Autodesk Inventor part; units mm, degrees
ref_plane "YZ Plane" through (0, 0, 0) normal (1, 0, 0) x (0, 1, 0)
ref_plane "XZ Plane" through (0, 0, 0) normal (0, 1, 0) x (-1, 0, 0)
ref_plane "XY Plane" through (0, 0, 0) normal (0, 0, 1) x (1, 0, 0)
sketch "Sketch1" plane through (0, 0, 0) normal (0, 0, 1) x (1, 0, 0)
  line L0 (-30, -40.5) -> (-30, 40.5)
  line L1 (-30, 40.5) -> (30, 40.5)
  line L2 (30, 40.5) -> (30, -40.5)
  line L3 (30, -40.5) -> (-30, -40.5)
  line L4 (-30, -40.5) -> (30, 40.5) construction
  line L5 (-30, 40.5) -> (30, -40.5) construction
  line L6 (-30, 40.5) -> (-10, 40.5)
  line L7 (-10, 40.5) -> (-10, 43.5)
  line L8 (-10, 43.5) -> (-30, 43.5)
  line L9 (-30, 43.5) -> (-30, 40.5) construction
  line L10 (30, 40.5) -> (10, 40.5)
  line L11 (10, 40.5) -> (10, 43.5)
  line L12 (10, 43.5) -> (30, 43.5)
  line L13 (30, 43.5) -> (30, 40.5)
  line L14 (-45.6, 0) -> (42.6, 0)
  line L15 (0, -60.9) -> (0, 60.9)
  line L16 (-10, -40.5) -> (-10, -43.5)
  line L17 (-10, -43.5) -> (-30, -43.5)
  line L18 (-30, -43.5) -> (-30, -40.5) construction
  line L19 (10, -40.5) -> (10, -43.5)
  line L20 (10, -43.5) -> (30, -43.5)
  line L21 (30, -43.5) -> (30, -40.5)
  line L22 (-30, -40.5) -> (-30, -24.3)
  line L23 (-30, -24.3) -> (-33, -24.3)
  line L24 (-33, -24.3) -> (-33, -40.5)
  line L25 (-33, -40.5) -> (-30, -40.5) construction
  line L26 (-30, -8.1) -> (-30, 8.1)
  line L27 (-30, 8.1) -> (-33, 8.1)
  line L28 (-33, 8.1) -> (-33, -8.1)
  line L29 (-33, -8.1) -> (-30, -8.1)
  line L30 (-30, 40.5) -> (-30, 24.3)
  line L31 (-30, 24.3) -> (-33, 24.3)
  line L32 (-33, 24.3) -> (-33, 40.5)
  line L33 (-33, 40.5) -> (-30, 40.5) construction
  line L34 (-30, 43.5) -> (-33, 43.5)
  line L35 (-33, 43.5) -> (-33, 40.5)
  line L36 (-30, -43.5) -> (-33, -43.5)
  line L37 (-33, -43.5) -> (-33, -40.5)
  point P0 (0, 0)
  point P1 (20, 43.5)
  point P2 (-20, 43.5)
  point P3 (20, -43.5)
  point P4 (-20, -43.5)
  point P5 (-33, 32.4)
  point P6 (-33, 0)
  point P7 (-33, -32.4)
  point P8 (-30, 0)
  dimension "d0" = 81
  dimension "d1" = 60
  dimension "d4" = 20
  dimension "d5" = 20
  dimension "d6" = 3
  dimension "d7" = 3
  dimension "d8" = 16.2
extrude "Extrusion1" add sketch "Sketch1" along normal blind 3
sketch "Sketch2" plane through (0, 0, 3) normal (0, 0, 1) x (1, 0, 0)
  line L0 (-45.6, 0) -> (42.6, 0)
  line L1 (0, -60.9) -> (0, 60.9)
  circle A0 centre (15, 0) radius 3.05
  line L2 (30, -43.5) -> (30, 43.5)
  dimension "d9" = 6.1
  dimension "d12" = 15
extrude "Extrusion2" cut sketch "Sketch2" against normal through all
equation "\"d4\" = 0.333333 * d1"
equation "\"d5\" = d4"
equation "\"d6\" = d2"
equation "\"d7\" = d2"
equation "\"d8\" = 0.2 * d0"
properties part number "top switch"
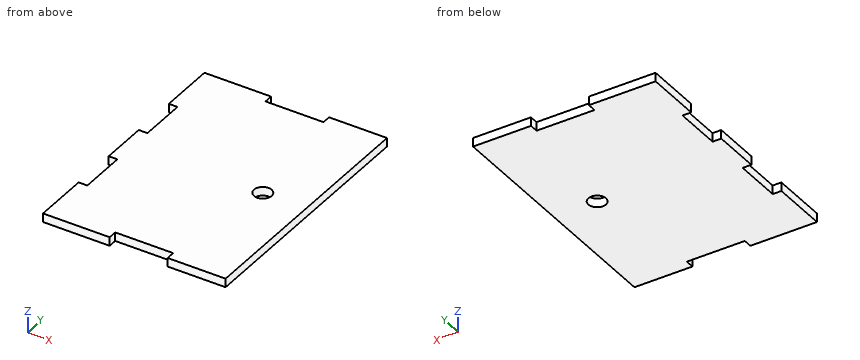
The listing builds one solid part. Answer for the finished solid, in the listing's coordinates (mm). Coordinates: 2 decimals unless noted, no trailing zeros. Write each loop counter-clockwise with the first axis right and the second up, starting at its lowest first coordinate (ties: lowest second). Pieces come first, ordered by that corner, then holes. Notation, with made-up numbers: M 86,-39.5 L 124,-39.5 A35 ccw 124,-5.5 Z; hole C 83.5,48 d10. An arc over 180 degrees is marked long. Put each result on its own line as item: value. Start each with the question number.
1. Consider line 1 (Y direction, x = 15, z = 2.15); line 2 (X direction, y = 0, z = 2); line 3 (Y direction, x = 0.5, z = 2.3). Determine where each line is inside the solid, lowest interval first. Write a range as from..to.
2. A cutting plane is placed at D-D on y = -18.5. Write down the section's boundary in (x, z), then the cut area to 3 significant figures.
3. A cutting plane is placed at B-B on y = 0. Write down the section's boundary in (x, z).
4. A cutting plane is placed at C-C on z = 1.85. Write down the section's boundary in (x, y), then the cut area to 3 significant figures.
5. A cutting plane is placed at A-A on x = 15. Write down the section's boundary in (y, z).
6. Flat-ended cylindrical pins translate along their axes: P1, Ø10, axis at x = 15, y = 0, coming from the +Z side; P2, Ø1.5, axis at y = 17, z = 1.5, coming from the -X side; P3, Ø1, axis at x = 4.5, z = 2.5, coming from the -Y side. Find the tip coordinate at first contact, or state that the pin passes through.
Resolved:
1. line 1: y = -43.5..-3.05, 3.05..43.5
1. line 2: x = -33..11.95, 18.05..30
1. line 3: y = -40.5..40.5
2. outline: M -30,0 L 30,0 L 30,3 L -30,3 Z
2. area: 180 mm2
3. outline: M -33,0 L 11.95,0 L 11.95,3 L -33,3 Z; M 18.05,0 L 30,0 L 30,3 L 18.05,3 Z
4. outline: M -33,-43.5 L -10,-43.5 L -10,-40.5 L 10,-40.5 L 10,-43.5 L 30,-43.5 L 30,43.5 L 10,43.5 L 10,40.5 L -10,40.5 L -10,43.5 L -33,43.5 L -33,24.3 L -30,24.3 L -30,8.1 L -33,8.1 L -33,-8.1 L -30,-8.1 L -30,-24.3 L -33,-24.3 Z; hole C 15,0 d6.1
4. area: 5,230 mm2
5. outline: M -43.5,0 L -3.05,0 L -3.05,3 L -43.5,3 Z; M 3.05,0 L 43.5,0 L 43.5,3 L 3.05,3 Z
6. P1: stops at z = 3
6. P2: stops at x = -30
6. P3: stops at y = -40.5
